Build history of the part. All positions in model axes, mm. Coordinates: 2 decimals unless noted, no trailing zeros. Order: outer loops, then holes, each group sorted by start corner. A loop starts at its lowest first (then second) coordinate and runs counter-clockwise, first axis right, second up. Notation, with made-up numbers: (68, -22.75) -> (91, -22.75) arc R15 cw to (91, -9.75) -> close; hole circle Ø11 at (61.25, 52.25). An arc over 180 degrees is marked (long way). Write each question's results on one line, items separated by ' | '.
from build123d import *

# Parameters (mm, degrees)
BOSS_EXTRUDE1_DEPTH = 3.175
SKETCH2_R           = 5.715
SKETCH2_W           = 29.972
SKETCH2_H           = 8.79475
SKETCH2_W_2         = 9.144
SKETCH2_H_2         = 11.049
CUT_EXTRUDE1_DEPTH  = 5.4356
SKETCH3_W           = 1.905
SKETCH3_H           = 1.235097614
CUT_EXTRUDE2_DEPTH  = 57.808955425
SKETCH4_W           = 5.501032945
SKETCH4_H           = 1.016
SKETCH4_W_2         = 19.558
SKETCH4_W_3         = 7.3914
CUT_EXTRUDE3_DEPTH  = 57.808955425
SKETCH5_W           = 31.75
SKETCH5_H           = 0.635
SKETCH5_W_2         = 29.845
CUT_EXTRUDE4_DEPTH  = 57.808955425


with BuildPart() as part:
    # Sketch1 → Boss-Extrude1 (new body)
    with BuildSketch(Plane.XY):
        Polygon((-51.8414, 0), (-51.8414, 7.3152), (-48.9204, 7.3152), (-48.9204, 17.3482), (-41.529, 17.3482), (-41.529, 22.7838), (-9.779, 22.7838), (-9.779, 17.3482), (9.779, 17.3482), (9.779, 22.7838), (41.529, 22.7838), (41.529, 17.3482), (51.943, 17.3482), (51.943, 7.3152), (49.022, 7.3152), (49.022, 0), (49.022, -7.2898), (51.943, -7.2898), (51.943, -14.1478), (41.529, -14.1478), (41.529, -19.5834), (9.779, -19.5834), (9.779, -14.1478), (-9.779, -14.1478), (-9.779, -19.5834), (-41.529, -19.5834), (-41.529, -14.1478), (-48.9204, -14.1478), (-48.9204, -7.2898), (-51.8414, -7.2898), align=None)
    extrude(amount=BOSS_EXTRUDE1_DEPTH)

    # Sketch2 → Cut-Extrude1 (cut)
    with BuildSketch(Plane.XY.offset(3.175)):
        with Locations((40.894, 15.9766)):
            Circle(SKETCH2_R)
        with Locations((-33.9344, 4.695825)):
            Rectangle(SKETCH2_W, SKETCH2_H)
        with Locations((9.3218, 2.3876)):
            Rectangle(SKETCH2_W_2, SKETCH2_H_2)
    extrude(amount=-CUT_EXTRUDE1_DEPTH, mode=Mode.SUBTRACT)

    # Sketch3 → Cut-Extrude2 (cut, through all)
    with BuildSketch(Plane.XY.offset(3.175)):
        with Locations((40.5765, 22.166251193)):
            Rectangle(SKETCH3_W, SKETCH3_H)
    extrude(amount=-CUT_EXTRUDE2_DEPTH, mode=Mode.SUBTRACT)

    # Sketch4 → Cut-Extrude3 (cut, through all)
    with BuildSketch(Plane.XY.offset(3.175)):
        with Locations((49.192483528, 16.8402)):
            Rectangle(SKETCH4_W, SKETCH4_H)
        with Locations((0, 16.8402)):
            Rectangle(SKETCH4_W_2, SKETCH4_H)
        with Locations((-45.2247, 16.8402)):
            Rectangle(SKETCH4_W_3, SKETCH4_H)
    extrude(amount=-CUT_EXTRUDE3_DEPTH, mode=Mode.SUBTRACT)

    # Sketch5 → Cut-Extrude4 (cut, through all)
    with BuildSketch(Plane.XY.offset(3.175)):
        with Locations((-25.654, 22.4663)):
            Rectangle(SKETCH5_W, SKETCH5_H)
        with Locations((24.7015, 22.4663)):
            Rectangle(SKETCH5_W_2, SKETCH5_H)
    extrude(amount=-CUT_EXTRUDE4_DEPTH, mode=Mode.SUBTRACT)


solid = part.part
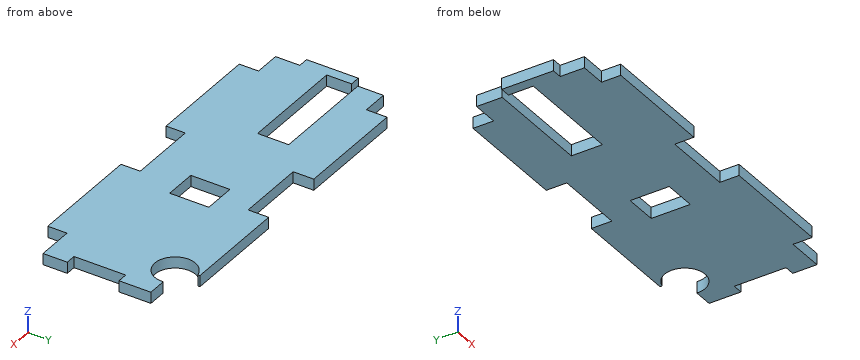
Item 1: Slice it at A-A, the plane x = -20. List the corners of the cut face in (y, z) (3 decimals), and give its area (3 significant figures).
Answer:
outline: (-19.583, 0) -> (0.298, 0) -> (0.298, 3.175) -> (-19.583, 3.175) -> close; (9.093, 0) -> (22.149, 0) -> (22.149, 3.175) -> (9.093, 3.175) -> close | area: 105 mm^2
Item 2: Slice it at C-C, the plane x = -4. List the corners of the cut face in (y, z) (3 decimals), and give its area (3 significant figures).
Answer:
outline: (-14.148, 0) -> (16.332, 0) -> (16.332, 3.175) -> (-14.148, 3.175) -> close | area: 96.8 mm^2
Item 3: Slice it at D-D, the plane y = -13. List the corners of the cut face in (x, z) (3 decimals), and give its area (3 significant figures).
Answer:
outline: (-48.92, 0) -> (51.943, 0) -> (51.943, 3.175) -> (-48.92, 3.175) -> close | area: 320 mm^2
Item 4: Drill centre lines: line 1 (X direction, y = 5, z = 2.45); line 2 (Y direction, x = -41, z = 2.5); line 3 (X direction, y = -2, z = 2.7). Where is each one in solid material? Low to high. Write a range as from..to.
Answer:
line 1: x = -51.84..-48.92, -18.95..4.75, 13.89..49.02 | line 2: y = -19.58..0.3, 9.09..22.15 | line 3: x = -51.84..4.75, 13.89..49.02
Item 5: Slice it at B-B, the plane y = 4. List the corners of the cut face in (x, z) (3 decimals), and give its area (3 significant figures).
Answer:
outline: (-51.841, 0) -> (-48.92, 0) -> (-48.92, 3.175) -> (-51.841, 3.175) -> close; (-18.948, 0) -> (4.75, 0) -> (4.75, 3.175) -> (-18.948, 3.175) -> close; (13.894, 0) -> (49.022, 0) -> (49.022, 3.175) -> (13.894, 3.175) -> close | area: 196 mm^2
Item 6: Pin check, flat tips, straight feed: pin 1 (1 mm diameter, centred on x = 49, z = 2, fed in from -Y); pin 2 (1 mm diameter, centred on y = 19.5, z = 1.5, fed in from -X); pin 3 (1.5 mm diameter, centred on y = 13, z = 3, fed in from -X). Stop position of each tip, or through.
Answer:
pin 1: stops at y = -14.15 | pin 2: stops at x = -41.53 | pin 3: stops at x = -48.92
